from build123d import *
from build123d.topology import SkipClean

# Parameters (mm, degrees)
SKETCH1_R           = 50
SKETCH1_R_2         = 45
BOSS_EXTRUDE1_DEPTH = 50
BOSS_EXTRUDE2_START = 5
SKETCH2_R           = 70
SKETCH2_R_2         = 45
BOSS_EXTRUDE2_DEPTH = 5
RIB1_START          = -2.5
RIB1_DEPTH          = 5
CIRPATTERN1_COUNT   = 8


# Read off the part's stored shape, not the designer's step: Rib1
with BuildPart() as part:
    # Sketch1 → Boss-Extrude1 (new body)
    with BuildSketch(Plane(origin=(0, 0, 0), x_dir=(1, 0, 0), z_dir=(0, 1, 0))):
        with Locations(Location((0, 0, 0), (0, 0, 270))):
            Circle(SKETCH1_R)
        with Locations(Location((0, 0, 0), (0, 0, 270))):
            Circle(SKETCH1_R_2, mode=Mode.SUBTRACT)
    extrude(amount=BOSS_EXTRUDE1_DEPTH)

    # Sketch2 → Boss-Extrude2 (add)
    with SkipClean():  # the faces are left unmerged after this step: merging them gives an invalid solid
        with BuildSketch(Plane.XZ.offset(BOSS_EXTRUDE2_START)):
            with Locations(Location((0, 0, 0), (0, 0, 270))):
                Circle(SKETCH2_R)
            with Locations(Location((0, 0, 0), (0, 0, 270))):
                Circle(SKETCH2_R_2, mode=Mode.SUBTRACT)
        extrude(amount=-BOSS_EXTRUDE2_DEPTH)

    # Rib1 outline → Rib1 (add)
    with SkipClean():  # the faces are left unmerged after this step: merging them gives an invalid solid
        with BuildSketch(Plane(origin=(0, 0, 0), x_dir=(0, 0, -1), z_dir=(1, 0, 0)).offset(RIB1_START)):
            Polygon((-48.219433675, 17), (-49.937460889, 15.281972786), (-65.219433674, 0), (-48, 0), (-48, 17), align=None)
        rib1 = extrude(amount=RIB1_DEPTH)
    add(part.part.scale(1), mode=Mode.REPLACE)  # the faces are merged on a copy

    # CirPattern1: Rib1 ×8 about axis
    cirpattern1_axis = Axis((0, 0, 0), (0, 1, 0))
    for i in range(1, CIRPATTERN1_COUNT):
        add(rib1.rotate(cirpattern1_axis, i * 360 / CIRPATTERN1_COUNT))


solid = part.part
Here's how the part is built. I have some questions about the finished solid (model axes, mm). A direction names the side the tool comes from. Round coordinates to 2 decimals unless told otherwise and drop trailing zeros. Order: outer loops, then holes, each group sorted by start corner. A loop starts at its lowest first (then second) coordinate and runs counter-clockwise, first axis right, second up. Notation, with made-up numbers: M 80.5,52.5 L 139.5,52.5 A17 cw 139.5,83.5 Z; hole C 53,27.25 d10. An arc over 180 degrees is marked long. One line per question, with ' | ' between items.
1) Imagine slicing it at B-B, the plane x = 0. Write out the boundary of the cut face in (y, z).
Checked values:
outline: M -5,-70 L 0,-70 L 0,-65.22 L 15.22,-50 L 50,-50 L 50,-45 L -5,-45 Z; M -5,45 L 50,45 L 50,50 L 15.22,50 L 0,65.22 L 0,70 L -5,70 Z
2) I'm going to push flat-ended pins straight in: pin 1 Ø7.5 at (x, y) = (57, 4.5) entering from +Z; pin 2 Ø7.5 at (y, z) = (6.5, 60.5) entering from -X; pin 3 Ø12 at (x, y) = (-25, 1) entering from +Z. Where does each tip first touch, or does it pass through?
Checked values:
pin 1: stops at z = 2.5 | pin 2: stops at x = -2.5 | pin 3: stops at z = 67.35
3) Imagine slicing it at A-A, the plane z = 12. Write out the boundary of the cut face in (x, y), plus the area to 3 significant figures.
Checked values:
outline: M -68.96,-5 L -43.37,-5 L -43.37,50 L -48.54,50 L -48.54,0 L -68.96,0 Z; M 43.37,-5 L 68.96,-5 L 68.96,0 L 48.54,0 L 48.54,50 L 43.37,50 Z | area: 773 mm²
4) We'd pull the mould along Y, two halves only. Please class faces 4 (the flat face through (-40.614, 7.748, -40.663)), 5 (the flat face through (-46, -5, 1)), 6 (the flat face through (36.621, 4.352, -40.156)): released by +Y, released by -Y, zero draft, split by the parting line, or undercut.
Checked values:
face 4: released by +Y | face 5: released by -Y | face 6: zero draft
5) I need wall thicknesses on line 1 (X direction, y = -2.7, z = 0); line 2 (Z direction, x = 0, y = 35). Which ranges of each line are inside material? Lowest first, please.
Checked values:
line 1: x = -70 to -45, 45 to 70 | line 2: z = -50 to -45, 45 to 50
6) Imagine slicing it at D-D, the plane z = -55. Write out the boundary of the cut face in (x, y).
Checked values:
outline: M -43.3,-5 L 43.3,-5 L 43.3,0 L 2.5,0 L 2.5,10.22 L -2.5,10.22 L -2.5,0 L -43.3,0 Z
7) On a 3-axis mill with a long thin cutter (end or side, diameter ignored), from which of +Z, -Z, +X, -X, +Y, -Y can I reach the whole of each face in a straight line? I mean faces 1 (the flat face through (40.156, 4.352, -36.621)), 2 (the flat face through (-54, 4, 2.5)), 3 (the flat face through (36.621, 4.352, 40.156)). Say none if no direction works.
Checked values:
face 1: +X, +Y | face 2: +Z, -X, +Y | face 3: +Z, +Y
